Input: dimensioned drawing with shaded views. Units: mm. Origin: part minimum x, y, z. Give positions to 0.01 mm unless a question says otherwise; leave off trailing zeros. Order: outer loops, then holes, each group sorted by start corner. A loop starts at its lowest first (then second) coordinate and runs counter-clockwise, first axis right, second up. Notation, with made-up numbers: M 81.25,42 L 109.25,42 A10 cw 109.25,50 Z; hole C 47.25,3 d8. An arc over 180 degrees is marked long. Answer in a Markdown table with one row per item. Add a question column.
(1) Mould query, pull axis Z, two halves, no side actions, for the marked faces 1, 2, 3 and 4. Classes: pulls with the +Z half, pulls with the -Z half, needs draft (parallel to the pull), parting line crosses it, or undercut.
(2) Pin query (flat end, axial travel): P1, Ø4, axis at x = 12.5, z = 7.5, coming from the -Y side; P2, Ø3, axis at y = 11.5, z = 12, coming from the -X side; P3, Ø1, axis at x = 3, z = 7, coming from the +Y side. Return the tip coordinate at first contact, or that it passes through.
(3) Material intervals for line 1 along Z through (x, y) = (16.75, 9.5) (1 decimal); line 2 along Z through (x, y) = (11, 11.75) (1 decimal); line 3 along Y through (x, z) = (21.25, 12), sorted ascending.
(4) Section query A-A, the plane y = 9.5. Return loops of the section in (x, z) (1 decimal).
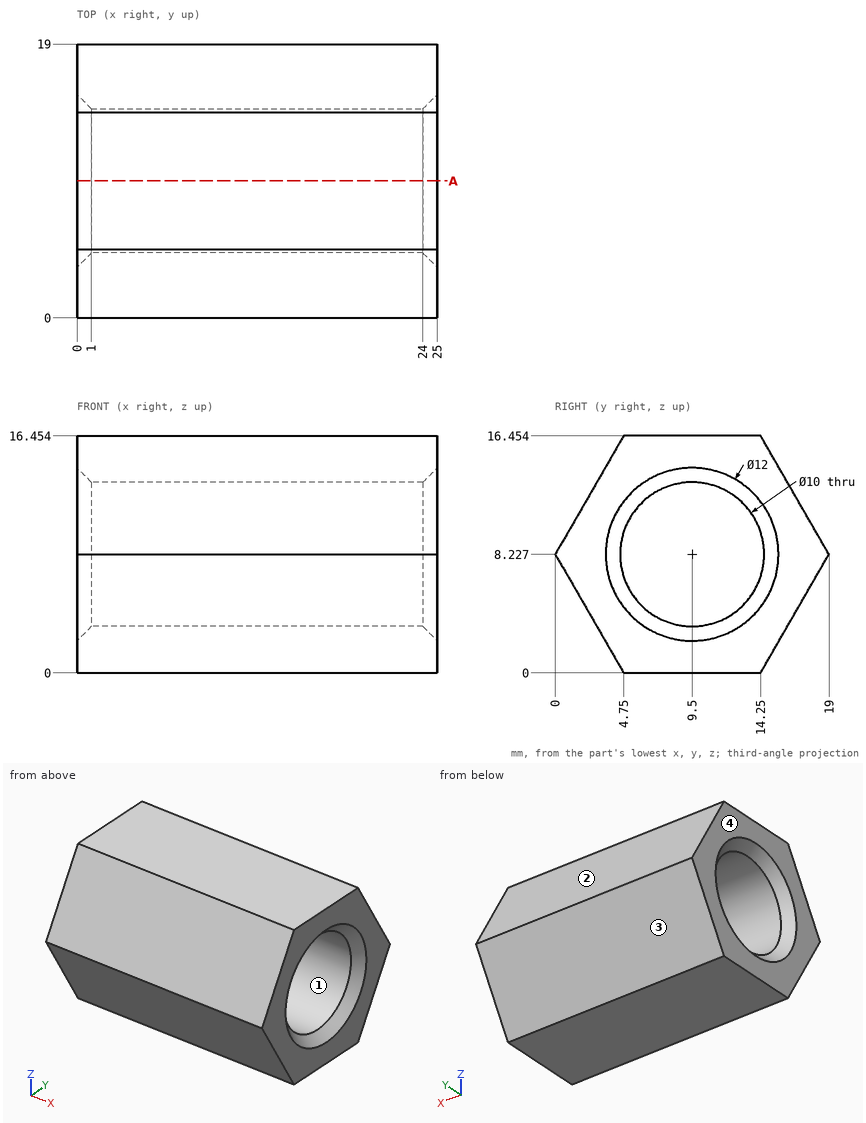
Values follow:
| question | item | result |
|---|---|---|
| 1 | face 1 | undercut |
| 1 | face 2 | pulls with the +Z half |
| 1 | face 3 | pulls with the -Z half |
| 1 | face 4 | needs draft |
| 2 | P1 | stops at y = 0 |
| 2 | P2 | stops at x = 0.23 |
| 2 | P3 | stops at y = 18.58 |
| 3 | line 1 | z = 0 to 3.2, 13.2 to 16.5 |
| 3 | line 2 | z = 0 to 3.8, 12.7 to 16.5 |
| 3 | line 3 | y = 2.18 to 6.22, 12.78 to 16.82 |
| 4 | outline | M 0,0 L 25,0 L 25,2.2 L 24,3.2 L 1,3.2 L 0,2.2 Z; M 0,14.2 L 1,13.2 L 24,13.2 L 25,14.2 L 25,16.5 L 0,16.5 Z |
